Build history of the part. All positions in model axes, mm. Face numbers are marked on the shaded views. A direction names the side the tool comes from. Give positions to 0.01 mm unless a question says otherwise; leave off trailing zeros. Write each loop counter-clockwise with the first axis right and the second up, starting at its lowest first coordinate (ties: lowest second). Pieces come first, ordered by that corner, then holes. Notation, with made-up numbers: (67.25, 89) -> (82.25, 89) arc R32 cw to (82.25, 119) -> close; hole circle Ø4 at (27.5, 85.5). An arc over 180 degrees is marked (long way). One line per question, with ' | ' between items. Start each with the question number.
(1) Pin check, flat tips, straight feed: P1, Ø1.2, axis at x = 0, y = -3.8, coming from the -Z side (3 decimals); P2, Ø1.5, axis at x = -4, y = -8, coming from the -Z side; P3, Ø3, axis at y = -8.5, z = 3, coming from the +X side; P4, Ø1, axis at x = 1, z = 2, coming from the -Y side. Stop position of each tip, or through.
(2) Band-saw the part on C-C, the plane z = 3.25. Give the cut face in (x, y), and give its area (3 significant figures).
(3) Band-saw the part on A-A, the plane x = 0. Give the cut face in (y, z), and give its area (3 significant figures).
(4) Drill centre lines: probe 1 along Y at (x, z) = (0, 2.5); probe 2 along X at (y, z) = (-11.25, 3.5); probe 3 along Y at (x, z) = (-2, 5.75). Where is each one in solid material? Low to high. Write a range as from..to.
(5) Pull direction Y, two halves, no side cores. Call the marked faces 4, 5 and 6: released by +Y, released by -Y, zero draft, split by the parting line, or undercut.
(6) Band-saw the part on B-B, the plane y = -3.8. Give the cut face in (x, z).
(7) Band-saw the part on D-D, the plane y = -9. Give the cut face in (x, z).
(8) Tool access for the marked faces 1, 2 and 3: list every direction of +Z, -Z, +X, -X, +Y, -Y with a clear straight run to the whole face (end or side of a thin tool).
from build123d import *

# Parameters (mm, degrees)
SKETCH1_W           = 13
SKETCH1_H           = 13
BOSS_EXTRUDE1_DEPTH = 6.5
SKETCH2_W           = 0.5
SKETCH2_H           = 3.5
BOSS_EXTRUDE2_DEPTH = 6.5
SKETCH3_R           = 1
CUT_EXTRUDE1_DEPTH  = 16.921683328
SKETCH4_R           = 1.5
BOSS_EXTRUDE3_DEPTH = 0.5


with BuildPart() as part:
    # Sketch1 → Boss-Extrude1 (new body)
    with BuildSketch(Plane.XY):
        Rectangle(SKETCH1_W, SKETCH1_H)
    extrude(amount=BOSS_EXTRUDE1_DEPTH)

    # Sketch2 → Boss-Extrude2 (add)
    with BuildSketch(Plane.XZ.offset(6.5)):
        with Locations((-3.25, 3.25)):
            Rectangle(SKETCH2_W, SKETCH2_H)
        with Locations((3.25, 3.25)):
            Rectangle(SKETCH2_W, SKETCH2_H)
    extrude(amount=BOSS_EXTRUDE2_DEPTH)

    # Sketch3 → Cut-Extrude1 (cut, through all)
    with BuildSketch(Plane.XY.offset(6.5)):
        with Locations((0, 3.8)):
            Circle(SKETCH3_R)
        with Locations((0, -3.8)):
            Circle(SKETCH3_R)
    extrude(amount=-CUT_EXTRUDE1_DEPTH, mode=Mode.SUBTRACT)

    # Sketch4 → Boss-Extrude3 (add)
    with BuildSketch(Plane(origin=(6.5, 0, 0), x_dir=(0, 0, -1), z_dir=(1, 0, 0))):
        with Locations(Location((-3.25, 0, 0), (0, 0, 270))):
            Circle(SKETCH4_R)
    extrude(amount=BOSS_EXTRUDE3_DEPTH)


solid = part.part
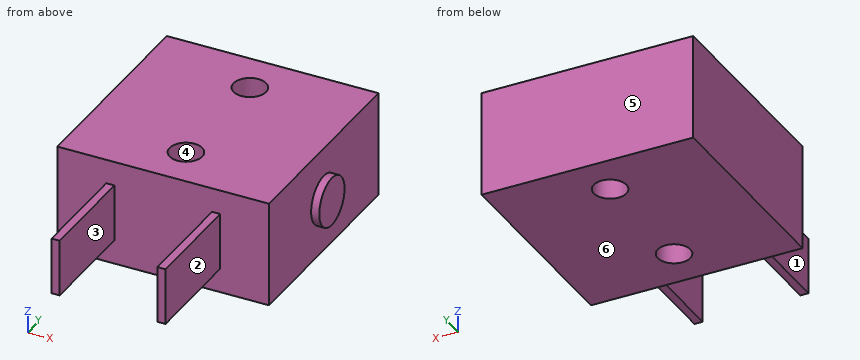
Results:
1) P1: passes through | P2: stops at z = 1.5 | P3: stops at x = 3.5 | P4: stops at y = -6.5
2) outline: (-6.5, -6.5) -> (-3.5, -6.5) -> (-3.5, -13) -> (-3, -13) -> (-3, -6.5) -> (3, -6.5) -> (3, -13) -> (3.5, -13) -> (3.5, -6.5) -> (6.5, -6.5) -> (6.5, -1.5) -> (7, -1.5) -> (7, 1.5) -> (6.5, 1.5) -> (6.5, 6.5) -> (-6.5, 6.5) -> close; hole circle Ø2 at (0, -3.8); hole circle Ø2 at (0, 3.8) | area: 171 mm²
3) outline: (-6.5, 0) -> (-4.8, 0) -> (-4.8, 6.5) -> (-6.5, 6.5) -> close; (-2.8, 0) -> (2.8, 0) -> (2.8, 6.5) -> (-2.8, 6.5) -> close; (4.8, 0) -> (6.5, 0) -> (6.5, 6.5) -> (4.8, 6.5) -> close | area: 58.5 mm²
4) probe 1: y = -6.5..-4.8, -2.8..2.8, 4.8..6.5 | probe 2: x = -3.5..-3, 3..3.5 | probe 3: y = -6.5..6.5
5) face 4: undercut | face 5: released by +Y | face 6: zero draft
6) outline: (-6.5, 0) -> (-1, 0) -> (-1, 6.5) -> (-6.5, 6.5) -> close; (1, 0) -> (6.5, 0) -> (6.5, 6.5) -> (1, 6.5) -> close
7) outline: (-3.5, 1.5) -> (-3, 1.5) -> (-3, 5) -> (-3.5, 5) -> close; (3, 1.5) -> (3.5, 1.5) -> (3.5, 5) -> (3, 5) -> close
8) face 1: +Z, -Z, -X, -Y | face 2: +Z, -Z, +X, -Y | face 3: +Z, -Z, -Y
